from build123d import *

# Parameters (mm, degrees)
F1_DEPTH = 70.3398883343
F3_R     = 7.3058881184
F3_R_2   = 9.1363164158
F4_DEPTH = 45
F5_W     = 23.752015084
F5_H     = 70.3398883343
F6_DEPTH = 20


with BuildPart() as f1:
    # F0 (on Front) → F1 (new body)
    with BuildSketch(Plane.XZ):
        with BuildLine():
            ThreePointArc((-36.1624062061, 20.6797644496), (-42.455005515, 46.4301466614), (-59.9144212902, 66.3762688637))
            Line((-59.9144212902, 66.3762688637), (-59.9144212902, -48.3024045825))
            Line((-59.9144212902, -48.3024045825), (-36.1624062061, -48.3024045825))
            Line((-36.1624062061, -48.3024045825), (-36.1624062061, 20.6797644496))
        make_face()
    extrude(amount=F1_DEPTH)

    # F3 (on face) → F4 (cut)
    with BuildSketch(Plane.XZ.offset(70.3398883343)):
        with Locations((-47.960318625, 28.4151956439)):
            Circle(F3_R)
        with Locations((-49.1870157421, -25.7221646607)):
            Circle(F3_R_2)
    extrude(amount=-F4_DEPTH, mode=Mode.SUBTRACT)

    # F5 (on face) → F6 (cut)
    with BuildSketch(Plane(origin=(0, 0, -48.3024045825), x_dir=(1, 0, 0), z_dir=(0, 0, -1))):
        with Locations((-48.0384137481, 35.1699441671)):
            Rectangle(F5_W, F5_H)
        Polygon((-42.0686118305, 10.4190278798), (-51.1485151947, 10.4190278798), (-55.7404533029, 27.6891775429), (-50.4079498351, 27.6891775429), (-50.4079498351, 53.3323399723), (-42.0686118305, 53.3323399723), align=None, mode=Mode.SUBTRACT)
    extrude(amount=-F6_DEPTH, mode=Mode.SUBTRACT)


solid = f1.part
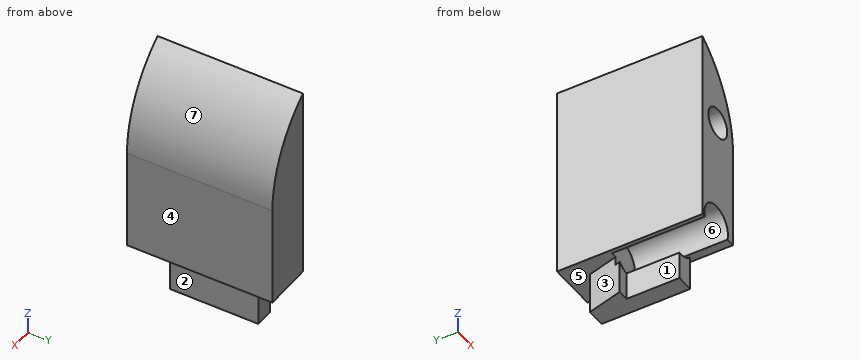
Geometry check sheet. Reference: the model listing, model coordinates, mm. Face numbers are marked on the shaded views. A direction names the side the tool comes from. Give positions to 0.01 mm unless a question says otherwise; leave off trailing zeros. Write each loop counter-clockwise with the first axis right and the second up, starting at its lowest first coordinate (ties: lowest second). Pieces come first, ordered by that corner, then holes.
1) Cross-section at A-A (y = -46.5). Record the boundary of the cut face in (x, z), plus the area to 3 significant figures.
Values follow:
outline: (-59.91, -28.3) - (-57.95, -28.3) arc R9.14 cw (long way) to (-40.42, -28.3) - (-36.16, -28.3) - (-36.16, 20.68) arc R55.83 ccw to (-59.91, 66.38) - close; (-50.41, -48.3) - (-42.07, -48.3) - (-42.07, -31.45) arc R9.14 cw to (-50.41, -34.78) - close; hole circle Ø14.61 at (-47.96, 28.42)
area: 1,700 mm2
2) Cross-section at B-B (x = -52.75). Record the boundary of the cut face in (y, z).
Values follow:
outline: (-70.34, -17.31) - (-25.34, -17.31) - (-25.34, -34.14) - (-27.69, -34.14) - (-27.69, -48.3) - (-16.44, -48.3) - (-16.44, -28.3) - (0, -28.3) - (0, 60.39) - (-70.34, 60.39) - (-70.34, 33.93) - (-25.34, 33.93) - (-25.34, 22.9) - (-70.34, 22.9) - close
3) Set-up check for the marked faces 1, 2, 3 and 4: record each of +Z, -Z, +X, -X, +Y, -Y from which the full face is reachable in a straight line by a thin tool's end or side.
Values follow:
face 1: -Z, -X, -Y
face 2: -Z, +X, +Y, -Y
face 3: -Z, -X, +Y
face 4: +Z, -Z, +X, +Y, -Y
4) Cross-section at D-D (z = 23). Record the boundary of the cut face in (x, y), plus the area to 3 significant figures.
Values follow:
outline: (-59.91, -70.34) - (-52.86, -70.34) - (-52.86, -25.34) - (-43.06, -25.34) - (-43.06, -70.34) - (-36.21, -70.34) - (-36.21, 0) - (-59.91, 0) - close
area: 1,230 mm2
5) Thickness scan on line 1 (Z direction, x = -45.5, y = -31); line 2 (Z direction, x = -46.75, y = -43); line 3 (Z direction, x = -44.5, y = -54). Record the ranges inside material, lowest first.
Values follow:
line 1: z = -48.3 to -34.08, -17.36 to 21.54, 35.29 to 51.59
line 2: z = -48.3 to -34.53, -16.92 to 21.21, 35.62 to 53.39
line 3: z = -17.88 to 21.98, 34.85 to 50.03
6) Go/stop test with flat-tipped pins: pin 1 Ø6 at (x, z) = (-52, -36.5) entering from -Y; pin 2 Ø7.5 at (x, z) = (-44.5, -43) entering from +Y; pin 3 Ø22 at (y, z) = (-24, -43) entering from +X. Record where each tip stops, or that it passes through.
Values follow:
pin 1: stops at y = -53.33
pin 2: stops at y = -10.42
pin 3: stops at x = -42.07
7) Cross-section at C-C (y = -61). Record the boundary of the cut face in (x, z).
Values follow:
outline: (-59.91, -28.3) - (-57.95, -28.3) arc R9.14 cw (long way) to (-40.42, -28.3) - (-36.16, -28.3) - (-36.16, 20.68) arc R55.83 ccw to (-59.91, 66.38) - close; hole circle Ø14.61 at (-47.96, 28.42)
8) Release check for a two-part mould opening along X. For the marked faces 5, 6 and 7 record: released by +X, released by -X, zero draft, split by the parting line, or undercut.
Values follow:
face 5: zero draft
face 6: undercut
face 7: released by +X
